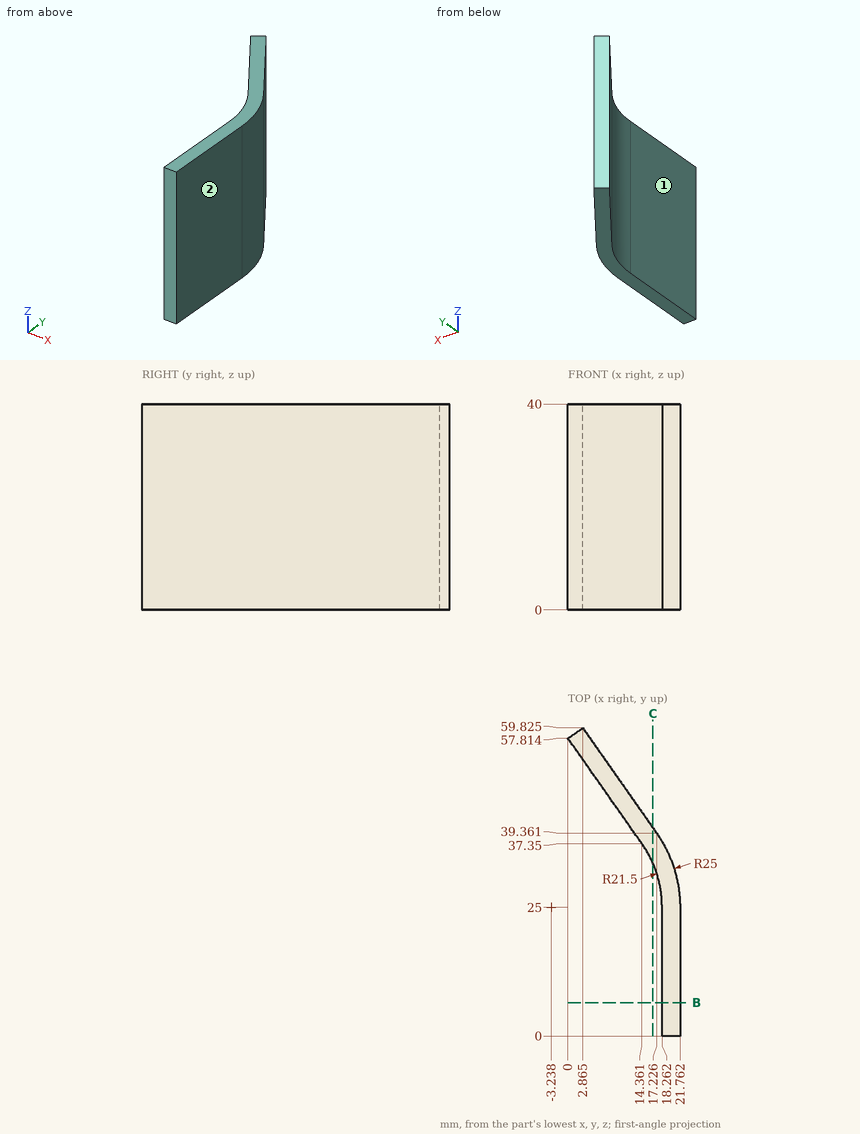
Check sheet for the drawn part. Datum: minimum x, y, z corner. Units: mm. A direction names the side the tool comes from. Coordinates: 2 decimals unless noted, no trailing zeros. Write each loop counter-clockwise with the first axis right and the second up, starting at its lowest first coordinate (ties: lowest second). Pieces come first, ordered by that corner, then holes. Notation, with made-up numbers: (-12, 63) - (5, 63) arc R18 ccw to (5, 80) - close; hole circle Ø1 at (63, 46). An arc over 180 degrees is marked (long way). Answer as a JSON object with one key per item and string values.
(1) Gauge pin test, flat ends, axial feed: pin 1 Ø1 at (x, z) = (17.5, 9) entering from +Y; pin 2 Ø10 at (y, z) = (32, 20) entering from +X; pin 3 Ø10 at (x, z) = (15.5, 34) entering from +Y (1 decimal); pin 4 Ø4 at (x, y) = (16, 8) entering from +Z. Record the tip position at first contact, or that the pin passes through.
Report:
{"pin 1": "y = 39.68", "pin 2": "x = 21.68", "pin 3": "y = 48.9", "pin 4": "through"}
(2) Cross-section at B-B on y = 6.5. Record the cut outline in (x, z).
Report:
{"outline": "(18.26, 0) - (21.76, 0) - (21.76, 40) - (18.26, 40) - close"}
(3) Cross-section at C-C on x = 16.5. Record the cut outline in (y, z) (1 decimal), plus the area to 3 significant figures.
Report:
{"outline": "(33.5, 0) - (40.4, 0) - (40.4, 40) - (33.5, 40) - close", "area": "275 mm^2"}
(4) Tool access check on the marked faces 1 and 2. Record the directions out of +Z, -Z, +X, -X, +Y, -Y that give a thin tool (end or side, any length) a straight path to the whole face; none if there is none.
Report:
{"face 1": "+Z, -Z, -X, -Y", "face 2": "+Z, -Z, +X, +Y, -Y"}
(5) Thickness scan on line 1 along X through (y, z) = (13.5, 21); line 2 along Y through (x, z) = (11.5, 21) (1 decimal); line 3 along Y through (x, z) = (4, 31) (1 decimal). Record the ranges inside material, lowest first.
Report:
{"line 1": "18.26 to 21.76", "line 2": "41.4 to 47.5", "line 3": "52.1 to 58.2"}
